Geometry: final body of the model. Coordinates: model frame, mm. A direction names the side the tool comes from. Give positions to 0.01 mm unless a question says otherwise; leave off trailing zeros. Write each loop counter-clockwise with the first axis right and the second up, starting at its lowest first coordinate (ties: lowest second). Pieces come first, ordered by that corner, then holes. Notation, with made-up numbers: (-30.75, 3.25) -> (-22.75, 3.25) arc R8 cw to (-22.75, 16.25) -> close; hole circle Ø11 at (-7.75, 2). An arc over 180 degrees is marked (long way). Answer in a Markdown table with one row per item. Add a question column.
Item 1: Section query C-C on x = -6.5. State how many separate pieces and enclosed holes the cut face has, plus the area to 3 significant figures.
Item 2: Section query A-A on z = 12. Output: boundary loops of the cut face in (x, y).
Item 3: Section query B-B on y = 42. Output: boundary loops of the cut face in (x, z), plus the area to 3 significant figures.
Item 4: Material intervals for probe 1 along Y at (x, z) = (-40, 1.25); probe 2 along Y at (x, z) = (-22.5, 11); probe 3 along Z at (x, y) = (-2.5, 10), sorted ascending. Write a range as from..to.
Item 5: Section query D-D on z = 20.5. Output: boundary loops of the cut face in (x, y).
Item 6: Access query for faces 4 (the flat face through (-14, 14, 0)), 5 (the flat face through (-7.77, 28.09, 9.42)), 6 (the cylindrical face through (-12.3, 11.9, 13.7)). Directions: +Z, -Z, +X, -X, +Y, -Y. A direction counts if a zero-diameter tool reaches every point of the face in a straight line with its end or side. Return the directions, or none.
Item 7: Draft query along Y for faces 1 (the flat face through (-14, 14, 24)), 2 (the cylindrical face through (-25.735, 4.405, 12.199)), 3 (the flat face through (-25, 25, 12)). Return one class per face: +Y half, -Y half, draft (parallel to the pull), parting line (faces both ways), or undercut.
Item 8: First-contact query: P1, Ø2, axis at y = 11.5, z = 12, coming from the +X side; P2, Ø2, axis at x = -15, z = 7.5, coming from the +Y side; P3, Ø5, axis at y = 14, z = 11, coming from the -X side. Flat tips, straight axial feed; report the tip coordinate or a pass-through.
```python
from build123d import *

# Parameters (mm, degrees)
F1_DEPTH = 24
F2_R     = 3.25
F3_DEPTH = 25
F4_START = -10
F2_R_2   = 6
F4_DEPTH = 15
F5_R     = 2
F6_DEPTH = 25


with BuildPart() as f1:
    # F0 (on Top) → F1 (new body)
    with BuildSketch(Plane.XY):
        Polygon((-50, 0), (0, 0), (0, 50), align=None)
    extrude(amount=F1_DEPTH)

    # F2 (on face) → F3 (cut)
    with BuildSketch(Plane(origin=(-25, 25, 0), x_dir=(-0.7071067812, -0.7071067812, 0), z_dir=(-0.7071067812, 0.7071067812, 0))):
        with Locations((-16.9469900429, 12)):
            Circle(F2_R)
        with Locations((21.0788715631, 12)):
            Circle(F2_R)
    extrude(amount=-F3_DEPTH, mode=Mode.SUBTRACT)

    # F2 (on face) → F4 (cut)
    with BuildSketch(Plane(origin=(-25, 25, 0), x_dir=(-0.7071067812, -0.7071067812, 0), z_dir=(-0.7071067812, 0.7071067812, 0)).offset(F4_START)):
        with Locations((21.0788715631, 12)):
            Circle(F2_R_2)
        with Locations((21.0788715631, 12)):
            Circle(F2_R, mode=Mode.SUBTRACT)
        with Locations((-16.9469900429, 12)):
            Circle(F2_R_2)
        with Locations((-16.9469900429, 12)):
            Circle(F2_R, mode=Mode.SUBTRACT)
    extrude(amount=-F4_DEPTH, mode=Mode.SUBTRACT)

    # F5 (on face) → F6 (cut)
    with BuildSketch(Plane.YZ):
        with Locations((10.8437594026, 12)):
            Circle(F5_R)
    extrude(amount=-F6_DEPTH, mode=Mode.SUBTRACT)


solid = f1.part
```
Findings below:
| question | item | result |
|---|---|---|
| 1 | separate pieces | 1 |
| 1 | enclosed holes | 2 |
| 1 | area | 934 mm^2 |
| 2 | outline | (-50, 0) -> (-35.86, 0) -> (-35.13, 0.73) -> (-42.2, 7.8) -> close; (-37.61, 12.39) -> (-30.54, 5.32) -> (-28.59, 7.27) -> (-21.32, 0) -> (0, 0) -> (0, 8.84) -> (-25, 8.84) -> (-25, 12.84) -> (0, 12.84) -> (0, 15.48) -> (-10.19, 25.67) -> (-8.24, 27.61) -> (-15.31, 34.69) -> close; (-10.72, 39.28) -> (-3.65, 32.21) -> (-1.7, 34.15) -> (0, 32.45) -> (0, 50) -> close |
| 3 | outline | (-8, 0) -> (0, 0) -> (0, 24) -> (-8, 24) -> close |
| 3 | area | 192 mm^2 |
| 4 | probe 1 | y = 0..10 |
| 4 | probe 2 | y = 1.06..9.11, 12.58..27.5 |
| 4 | probe 3 | z = 0..10.19, 13.81..24 |
| 5 | outline | (-50, 0) -> (0, 0) -> (0, 50) -> close |
| 6 | face 4 | -Z, +X, -X, +Y, -Y |
| 6 | face 5 | none |
| 6 | face 6 | +X |
| 7 | face 1 | draft |
| 7 | face 2 | undercut |
| 7 | face 3 | +Y half |
| 8 | P1 | stops at x = -25 |
| 8 | P2 | stops at y = 36 |
| 8 | P3 | stops at x = -38.2 |
